CAD build for the part. Positions are in the model's coordinates, mm. Round coordinates to 2 decimals unless told otherwise and drop trailing zeros. Order: outer loops, then holes, each group sorted by start corner. A loop starts at its lowest first (then second) coordinate and runs counter-clockwise, first axis right, second up. Notation, with made-up numbers: M 84,-26.75 L 120,-26.75 A33 cw 120,1.25 Z; hole C 78.25,-20 d3. An arc over 180 degrees is marked long. Put each result on its own line as item: value.
```python
from build123d import *

# Parameters (mm, degrees)
SKETCH_1_W             = 21
SKETCH_1_H             = 1
EXTRUDE_1_DEPTH        = 0.4
PATTERN_LINEAR_1_COUNT = 6
PATTERN_LINEAR_1_PITCH = 3
EXTRUDE_3_DEPTH        = 0.4
PATTERN_LINEAR_2_COUNT = 8
PATTERN_LINEAR_2_PITCH = 3


with BuildPart() as part:
    # Sketch 1 → Extrude 1 (new body)
    with BuildSketch(Plane.XY):
        with Locations((10.5, 0.5)):
            Rectangle(SKETCH_1_W, SKETCH_1_H)
    extrude(amount=EXTRUDE_1_DEPTH)


with BuildPart() as pattern_linear_1_1:
    # Pattern Linear 1: pattern copy
    add(part.part.moved(Location(Vector(0, 1, 0) * (1 * PATTERN_LINEAR_1_PITCH))))


with BuildPart() as pattern_linear_1_2:
    # Pattern Linear 1: pattern copy
    add(part.part.moved(Location(Vector(0, 1, 0) * (2 * PATTERN_LINEAR_1_PITCH))))


with BuildPart() as pattern_linear_1_3:
    # Pattern Linear 1: pattern copy
    add(part.part.moved(Location(Vector(0, 1, 0) * (3 * PATTERN_LINEAR_1_PITCH))))


with BuildPart() as pattern_linear_1_4:
    # Pattern Linear 1: pattern copy
    add(part.part.moved(Location(Vector(0, 1, 0) * (4 * PATTERN_LINEAR_1_PITCH))))


with BuildPart() as pattern_linear_1_5:
    # Pattern Linear 1: pattern copy
    add(part.part.moved(Location(Vector(0, 1, 0) * (5 * PATTERN_LINEAR_1_PITCH))))


with BuildPart() as part_1:
    add(part.part)

    add(pattern_linear_1_1.part)  # Extrude 3 merges Pattern Linear 1_1

    add(pattern_linear_1_2.part)  # Extrude 3 merges Pattern Linear 1_2

    add(pattern_linear_1_3.part)  # Extrude 3 merges Pattern Linear 1_3
    # Sketch 3 → Extrude 3 (add)
    with BuildSketch(Plane.XY.offset(0.4)):
        Polygon((0, 16), (0, 10), (0, 0), (-1, 0), (-1, 10.98507125), (-1, 16), align=None)
    extrude_3 = extrude(amount=-EXTRUDE_3_DEPTH)

    # Pattern Linear 2: Extrude 3 ×8
    with Locations(*[(i * PATTERN_LINEAR_2_PITCH, 0, 0) for i in range(1, PATTERN_LINEAR_2_COUNT)]):
        add(extrude_3)

    # Combine 1: read off the stored shape, not the designer's step
    # Combine 1: union Pattern Linear 1_4, Pattern Linear 1_5
    add(pattern_linear_1_4.part)
    add(pattern_linear_1_5.part)


solid = part_1.part
```
Item 1: Probe line 1 along Y through (x, z) = (16.5, 0.15). List the from-to ranges inside material, lowest first. Write a range as [from, to].
Answers below:
line 1: [0, 1], [3, 4], [6, 7], [9, 10], [12, 13], [15, 16]
Item 2: Band-saw the part on A-A on x = 16.75. Give the cut face in (y, z), and give its area (3 significant figures).
Answers below:
outline: M 0,0 L 1,0 L 1,0.4 L 0,0.4 Z; M 3,0 L 4,0 L 4,0.4 L 3,0.4 Z; M 6,0 L 7,0 L 7,0.4 L 6,0.4 Z; M 9,0 L 10,0 L 10,0.4 L 9,0.4 Z; M 12,0 L 13,0 L 13,0.4 L 12,0.4 Z; M 15,0 L 16,0 L 16,0.4 L 15,0.4 Z
area: 2.40 mm²
Item 3: Band-saw the part on B-B on y = 2.5. State how many separate pieces and enclosed holes the cut face has, and give its area (3 significant figures).
Answers below:
separate pieces: 8
enclosed holes: 0
area: 3.20 mm²
